```python
from build123d import *

# Parameters (mm, degrees)
SKETCH1_W           = 35
SKETCH1_H           = 30
SKETCH1_R           = 5
BOSS_EXTRUDE1_DEPTH = 20
SKETCH2_R           = 2.5
CUT_EXTRUDE1_DEPTH  = 44.011626335
SKETCH3_R           = 1.5
CUT_EXTRUDE2_DEPTH  = 47.165463282


with BuildPart() as part:
    # Sketch1 → Boss-Extrude1 (new, symmetric)
    with BuildSketch(Plane.XY):
        Rectangle(SKETCH1_W, SKETCH1_H)
        Circle(SKETCH1_R, mode=Mode.SUBTRACT)
    extrude(amount=BOSS_EXTRUDE1_DEPTH, both=True)

    # Sketch2 → Cut-Extrude1 (cut, through all)
    with BuildSketch(Plane(origin=(17.5, 0, 0), x_dir=(0, 0, -1), z_dir=(1, 0, 0))):
        with Locations((-15, 10)):
            Circle(SKETCH2_R)
        with Locations((15, 10)):
            Circle(SKETCH2_R)
        with Locations(Location((15, -10, 0), (0, 0, 180))):
            Circle(SKETCH2_R)
        with Locations(Location((-15, -10, 0), (0, 0, 180))):
            Circle(SKETCH2_R)
    extrude(amount=-CUT_EXTRUDE1_DEPTH, mode=Mode.SUBTRACT)

    # Sketch3 → Cut-Extrude2 (cut, through all)
    with BuildSketch(Plane.XY.offset(20)):
        with Locations((12, 0)):
            Circle(SKETCH3_R)
        with Locations((-12, 0)):
            Circle(SKETCH3_R)
    extrude(amount=-CUT_EXTRUDE2_DEPTH, mode=Mode.SUBTRACT)


solid = part.part
```
Build history of the part. All positions in model axes, mm. Give positions to 0.01 mm unless a question says otherwise; leave off trailing zeros. Order: outer loops, then holes, each group sorted by start corner. A loop starts at its lowest first (then second) coordinate and runs counter-clockwise, first axis right, second up. Notation, with made-up numbers: M -17.5,26.25 L 7.5,26.25 A33 ccw 7.5,58.25 Z; hole C 32.5,62 d3. An arc over 180 degrees is marked long. Return JSON: item names as keys, results as strings.
Q1. Band-saw the part on B-B (z = -15). Give the cut face in (x, y).
Answer list:
{"outline": "M -17.5,-15 L 17.5,-15 L 17.5,-12.5 L -17.5,-12.5 Z; M -17.5,-7.5 L 17.5,-7.5 L 17.5,7.5 L -17.5,7.5 Z; M -17.5,12.5 L 17.5,12.5 L 17.5,15 L -17.5,15 Z; hole C -12,0 d3; hole C 0,0 d10; hole C 12,0 d3"}
Q2. Band-saw the part on A-A (x = -12). Give the cut face in (y, z).
Answer list:
{"outline": "M -15,-20 L -1.5,-20 L -1.5,20 L -15,20 Z; M 1.5,-20 L 15,-20 L 15,20 L 1.5,20 Z; hole C -10,-15 d5; hole C -10,15 d5; hole C 10,-15 d5; hole C 10,15 d5"}
Q3. Band-saw the part on D-D (y = 0). Give the cut face in (x, z).
Answer list:
{"outline": "M -17.5,-20 L -13.5,-20 L -13.5,20 L -17.5,20 Z; M -10.5,-20 L -5,-20 L -5,20 L -10.5,20 Z; M 5,-20 L 10.5,-20 L 10.5,20 L 5,20 Z; M 13.5,-20 L 17.5,-20 L 17.5,20 L 13.5,20 Z"}
Q4. Band-saw the part on C-C (z = 3.5). Give the cut face in (x, y), then the cut area to 3 significant figures.
Answer list:
{"outline": "M -17.5,-15 L 17.5,-15 L 17.5,15 L -17.5,15 Z; hole C -12,0 d3; hole C 0,0 d10; hole C 12,0 d3", "area": "957 mm^2"}
Q5. Two-plate mould, pull along X, no slides. Class faces 1 (the face through (10.5, 0.07, 0.28)), 2 (the face through (17.5, 0, 0)), 3 (the face through (-4, 4, 20)), 4 (the face through (-13.5, 0.07, 0.28)): pulls with the +X half, pulls with the -X half, needs draft (parallel to the pull), parting line crosses it, or undercut.
Answer list:
{"face 1": "undercut", "face 2": "pulls with the +X half", "face 3": "needs draft", "face 4": "undercut"}
Q6. Wall check: probe 1 along Y at (x, z) = (0, 3.5); probe 2 along Z at (x, y) = (-3, 10.5); probe 3 along Y at (x, z) = (-2, -16.5). Give the ranges that are in metal, low to high. Write a range as from..to.
Answer list:
{"probe 1": "y = -15..-5, 5..15", "probe 2": "z = -20..-17.45, -12.55..12.55, 17.45..20", "probe 3": "y = -15..-12, -8..-4.58, 4.58..8, 12..15"}
